For this review, use the dimensioned drawing (mm, ordinates from the lowest corner) and the shaded views. A direction names the side the tool comes from. Give positions to 0.01 mm unless a question says otherwise; leave off trailing zeros. Write each loop counter-clockwise with the first axis right and the second up, starting at its lowest first coordinate (ties: lowest second). Pieces come first, ordered by that corner, then holes. Notation, with made-up numbers: (28.5, -30) -> (41.5, -30) arc R22 cw to (41.5, 2) -> close; hole circle Ø10 at (-23, -31). An arc over 180 degrees is marked (long way). Write each question's results on one line, items separated by ' | '. Start each with the question number.
(1) For the marked faces 1 and 2, list the 3-axis set-ups (+Z, -Z, +X, -X, +Y, -Y) from which the entire face can be reached by the end or side of a thin tool; tool diameter is ignored.
(2) To check wall thickness, follow probe 1 along Y at (x, z) = (2.25, 15); probe 2 along X at (y, z) = (3.25, 15); probe 3 along Y at (x, z) = (27.5, 20.5). State the ranges of each line that lie inside material, in increasing order.
(3) Take a section at B-B (z = 15). State the section outline as (x, y) points.
(4) Take a section at A-A (y = 46.5). State the section outline as (x, z) points, plus the area to 3 significant figures.
(5) Take a section at D-D (z = 19.75). State the section outline as (x, y) points, plus the area to 3 significant figures.
(6) Clearance check with flat-ended pins moving along their axes: pin 1 (4 mm diameter, centred on y = 19, z = 7, fed in from +X); pin 2 (3.5 mm diameter, centred on x = 22.5, z = 15, fed in from -Y); pin 3 (10 mm diameter, centred on x = 26, z = 17, fed in from +Y). State where each tip first meets the part, or that it passes through.
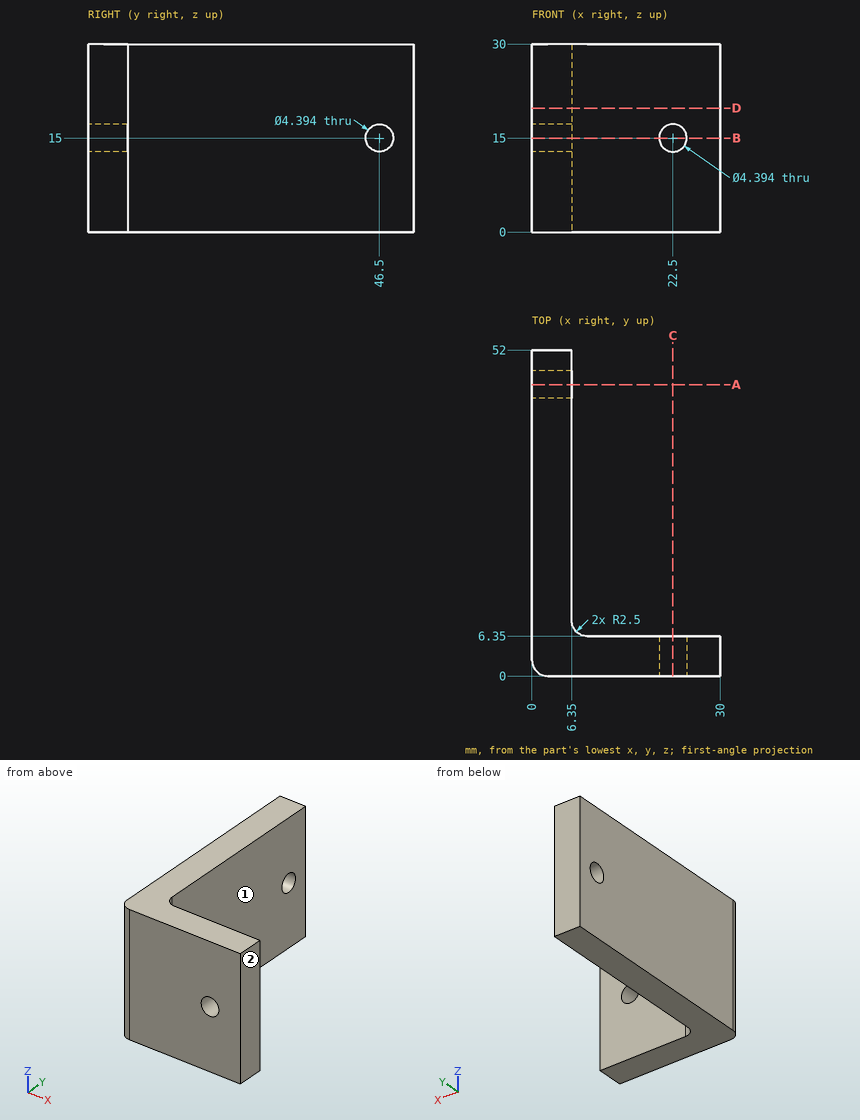
Report:
1) face 1: +Z, -Z, +X, +Y | face 2: +Z, -Z, +X, +Y, -Y
2) probe 1: 0.01 to 44.3, 48.7 to 52 | probe 2: 0 to 20.3, 24.7 to 30 | probe 3: 0 to 6.35
3) outline: (0, 2.5) arc R2.5 ccw to (2.5, 0) -> (20.3, 0) -> (20.3, 6.35) -> (8.85, 6.35) arc R2.5 cw to (6.35, 8.85) -> (6.35, 44.3) -> (0, 44.3) -> close; (0, 48.7) -> (6.35, 48.7) -> (6.35, 52) -> (0, 52) -> close; (24.7, 0) -> (30, 0) -> (30, 6.35) -> (24.7, 6.35) -> close
4) outline: (0, 0) -> (6.35, 0) -> (6.35, 12.8) -> (0, 12.8) -> close; (0, 17.2) -> (6.35, 17.2) -> (6.35, 30) -> (0, 30) -> close | area: 163 mm2
5) outline: (0, 2.5) arc R2.5 ccw to (2.5, 0) -> (30, 0) -> (30, 6.35) -> (8.85, 6.35) arc R2.5 cw to (6.35, 8.85) -> (6.35, 52) -> (0, 52) -> close | area: 480 mm2
6) pin 1: x = 6.35 | pin 2: through | pin 3: y = 6.35
